from build123d import *

# Parameters (mm, degrees)
CROQUIS1_W              = 190
CROQUIS1_H              = 120
CROQUIS1_R              = 2.25
CROQUIS1_R_2            = 5
CROQUIS1_R_3            = 1.25
SALIENTE_EXTRUIR1_DEPTH = 5


with BuildPart() as part:
    # Croquis1 → Saliente-Extruir1 (new body)
    with BuildSketch(Plane.XY):
        with Locations((-34.5, 32.5)):
            Rectangle(CROQUIS1_W, CROQUIS1_H)
        with Locations((36.5, 32.5)):
            Circle(CROQUIS1_R, mode=Mode.SUBTRACT)
        with Locations((-91.623199077, 0.069259856)):
            Circle(CROQUIS1_R, mode=Mode.SUBTRACT)
        with Locations((-91.623199077, 64.930740144)):
            Circle(CROQUIS1_R, mode=Mode.SUBTRACT)
        with Locations((-66.5, 62.5)):
            Circle(CROQUIS1_R_2, mode=Mode.SUBTRACT)
        with Locations((-6.5, 62.5)):
            Circle(CROQUIS1_R_2, mode=Mode.SUBTRACT)
        with Locations((-6.5, 6.5)):
            Circle(CROQUIS1_R_2, mode=Mode.SUBTRACT)
        with Locations((-66.5, 6.5)):
            Circle(CROQUIS1_R_2, mode=Mode.SUBTRACT)
        with Locations((-54.5, 50.5)):
            Circle(CROQUIS1_R_3, mode=Mode.SUBTRACT)
        with Locations((-18.5, 50.5)):
            Circle(CROQUIS1_R_3, mode=Mode.SUBTRACT)
        with Locations((-18.5, 18.5)):
            Circle(CROQUIS1_R_3, mode=Mode.SUBTRACT)
        with Locations((-54.5, 18.5)):
            Circle(CROQUIS1_R_3, mode=Mode.SUBTRACT)
    extrude(amount=SALIENTE_EXTRUIR1_DEPTH)


solid = part.part
The model under review builds one solid part; all positions refer to its coordinate system, in mm. Coordinates: 2 decimals unless noted, no trailing zeros. Write each loop counter-clockwise with the first axis right and the second up, starting at its lowest first coordinate (ties: lowest second). Pieces come first, ordered by that corner, then holes. Notation, with made-up numbers: (-2, 61) - (56, 61) arc R18 cw to (56, 86) - close; hole circle Ø3 at (46.5, -0.75). An arc over 180 degrees is marked (long way). Answer as a JSON object with one key per item and string values. Group by question number.
1. To check wall thickness, follow probe 1 along Y at (x, z) = (-6.5, 3.9); probe 2 along Y at (x, z) = (-54.5, 3.6); probe 3 along X at (y, z) = (9, 0.7). State the ranges of each line that lie inside material, in increasing order.
2. Mouldability with a two-part tool opening along Y and no side actions: class faces 1 (the face through (-93.87, 0.17, 2.46)), 2 (the face through (-36, 92.5, 2)), 3 (the face through (-129.5, 32, 2)) as pulls with the +Y half, pulls with the -Y half, needs draft (parallel to the pull), parting line crosses it, or undercut.
3. Add section D-D (z = 2.45). Give the number of separate pieces and of enclosed holes in the cut face, plus the area to 3 significant figures.
4. Clearance check with a flat-ended pin moving along its axis: pin 1 Ø9 at (x, y) = (-66.5, 62.5) entering from -Z. State where the tip first meets the part, or that it passes through.
5. Add section B-B (y = 32.5). Give the boundary of the cut face in (x, z), plus the area to 4 significant figures.
6. Add section A-A (x = 36.5). Give the boundary of the cut face in (y, z), plus the area to 4 significant figures.
7. Add section C-C (x = -6.5). Give the boundary of the cut face in (y, z), plus the area to 3 significant figures.
Findings:
{
 "1": {"probe 1": "-27.5 to 1.5, 11.5 to 57.5, 67.5 to 92.5", "probe 2": "-27.5 to 17.25, 19.75 to 49.25, 51.75 to 92.5", "probe 3": "-129.5 to -70.83, -62.17 to -10.83, -2.17 to 60.5"},
 "2": {"face 1": "undercut", "face 2": "pulls with the +Y half", "face 3": "needs draft"},
 "3": {"separate pieces": "1", "enclosed holes": "11", "area": "22,400 mm²"},
 "4": {"pin 1": "through"},
 "5": {"outline": "(-129.5, 0) - (34.25, 0) - (34.25, 5) - (-129.5, 5) - close; (38.75, 0) - (60.5, 0) - (60.5, 5) - (38.75, 5) - close", "area": "927.5 mm²"},
 "6": {"outline": "(-27.5, 0) - (30.25, 0) - (30.25, 5) - (-27.5, 5) - close; (34.75, 0) - (92.5, 0) - (92.5, 5) - (34.75, 5) - close", "area": "577.5 mm²"},
 "7": {"outline": "(-27.5, 0) - (1.5, 0) - (1.5, 5) - (-27.5, 5) - close; (11.5, 0) - (57.5, 0) - (57.5, 5) - (11.5, 5) - close; (67.5, 0) - (92.5, 0) - (92.5, 5) - (67.5, 5) - close", "area": "500 mm²"}
}
